Read the model definition and answer for the solid it produces. Units are mm, in the model's axes. Coordinates: 2 decimals unless noted, no trailing zeros. Loops run counter-clockwise (first coordinate to the right, second up) from the corner with the lowest first, then second, coordinate; pieces in that order, holes last. Notation, with made-up numbers: (-24, -27) - (-14, -27) arc R25 ccw to (-14, -7) - close; hole circle Ø1 at (-28, -2.5). An arc over 180 degrees is marked (long way). Use one line per item in the form item = value.
from build123d import *

# Parameters (mm, degrees)
F0_W           = 279.4
F0_H           = 101.6
F1_DEPTH       = 12.7
F2_D           = 6.35
F2_CSINK_D     = 12.7
F2_CSINK_ANGLE = 82
F3_D           = 7.9375
F4_R           = 12.7


with BuildPart() as f1:
    # F0 (on Front) → F1 (new body)
    with BuildSketch(Plane.XZ):
        with Locations((0, -50.8)):
            Rectangle(F0_W, F0_H)
    extrude(amount=F1_DEPTH)

    # F2 (through all)
    with Locations(Plane(origin=(0, 0, 0), x_dir=(1, 0, 0), z_dir=(0, 1, 0))):
        with Locations((-128.5875, 50.8), (128.5875, 50.8)):
            CounterSinkHole(F2_D / 2, F2_CSINK_D / 2, counter_sink_angle=F2_CSINK_ANGLE)

    # F3 (through all)
    with Locations(Plane(origin=(0, 0, 0), x_dir=(1, 0, 0), z_dir=(0, 1, 0))):
        with Locations((-101.6, 50.8), (0, 50.8)):
            Hole(F3_D / 2)

    # F4
    f4_edges = [f1.edges().sort_by_distance(p)[0] for p in [
        (139.7, -6.35, 0),
        (139.7, -6.35, -101.6),
        (-139.7, -6.35, -101.6),
        (-139.7, -6.35, 0),
    ]]
    fillet(f4_edges, radius=F4_R)


solid = f1.part
Item 1: Each of these flat-tipped pins is pushed along its axis until it touches: P1, Ø5.5, axis at x = -128.59, z = -50.8, coming from the +Y side; P2, Ø1, axis at x = 86, z = -36.5, coming from the +Y side; P3, Ø8.5, axis at x = 128.59, z = -50.8, coming from the +Y side. Where does it stop, or does it pass through?
Results below:
P1 = through
P2 = 0
P3 = -2.41
Item 2: The part is cut by section B-B on z = -50.8. Give the vertices of the cut face in (x, y), plus the area to 3 significant figures.
Results below:
outline = (-139.7, -12.7) - (-131.76, -12.7) - (-131.76, -3.65) - (-134.94, 0) - (-139.7, 0) - close; (-125.41, -12.7) - (-105.57, -12.7) - (-105.57, 0) - (-122.24, 0) - (-125.41, -3.65) - close; (-97.63, -12.7) - (-3.97, -12.7) - (-3.97, 0) - (-97.63, 0) - close; (3.97, -12.7) - (125.41, -12.7) - (125.41, -3.65) - (122.24, 0) - (3.97, 0) - close; (131.76, -12.7) - (139.7, -12.7) - (139.7, 0) - (134.94, 0) - (131.76, -3.65) - close
area = 3,160 mm²
Item 3: For a pull along Z with two mould halves and no side action, classify faces 1 (the flat face through (-139.7, -6, -51)), 2 (the cylindrical face through (-97.635, -6.439, -50.974)), 3 (the conical face through (125.412, -3.475, -51.8)), 4 (the flat face through (-2, -6, -101.6)) as +Z half, -Z half, draft (parallel to the pull), parting line (faces both ways), or undercut.
Results below:
face_1 = draft
face_2 = undercut
face_3 = undercut
face_4 = -Z half
Item 4: Find the intervals of material crossed by L1, parallel to X at y = -9.25, z = -50.8; L2, parallel to Z at x = 0, y = -8.25; L3, parallel to Z at x = -104.5, y = -10, in increasing order.
Results below:
L1 = -139.7 to -131.76, -125.41 to -105.57, -97.63 to -3.97, 3.97 to 125.41, 131.76 to 139.7
L2 = -101.6 to -54.77, -46.83 to 0
L3 = -101.6 to -53.51, -48.09 to 0
Item 5: The part is cut by section A-A on x = 0. Give the vertices of the cut face in (y, z).
Results below:
outline = (-12.7, -101.6) - (0, -101.6) - (0, -54.77) - (-12.7, -54.77) - close; (-12.7, -46.83) - (0, -46.83) - (0, 0) - (-12.7, 0) - close
